```python
from build123d import *

# Parameters (mm, degrees)
SKIZZE2_W                        = 120
SKIZZE2_H                        = 39.364160046
AUFSATZ_LINEAR_AUSTRAGEN1_DEPTH  = 30
SKIZZE24_R                       = 1.55
SCHNITT_LINEAR_AUSTRAGEN4_DEPTH  = 130.805766806
SKIZZE46_R                       = 2.85
SCHNITT_LINEAR_AUSTRAGEN15_DEPTH = 10
SCHNITT_LINEAR_START             = -5
SCHNITT_LINEAR_AUSTRAGEN25_DEPTH = 2.7
LINEARES_MUSTER1_COUNT           = 5
LINEARES_MUSTER1_PITCH           = 20
SPIEGELN2_COPY_1_SKETCH_R        = 2.85
SPIEGELN2_COPY_1_DEPTH           = 10
SPIEGELN2_COPY_2_SKETCH_R        = 2.85
SPIEGELN2_COPY_2_DEPTH           = 10
SPIEGELN2_COPY_3_SKETCH_R        = 2.85
SPIEGELN2_COPY_3_DEPTH           = 10
SPIEGELN2_COPY_4_SKETCH_R        = 2.85
SPIEGELN2_COPY_4_DEPTH           = 10
SPIEGELN2_START                  = -5
SPIEGELN2_COPY_5_DEPTH           = 2.7
SPIEGELN2_COPY_6_DEPTH           = 2.7
SPIEGELN2_COPY_7_DEPTH           = 2.7
SPIEGELN2_COPY_8_DEPTH           = 2.7
SKIZZE51_R                       = 1.55
SCHNITT_LINEAR_AUSTRAGEN26_DEPTH = 130.805766806
SKIZZE67_R                       = 0.5
SCHNITT_LINEAR_AUSTRAGEN28_DEPTH = 16
SKIZZE68_R                       = 0.65
SCHNITT_LINEAR_AUSTRAGEN30_DEPTH = 16
SKIZZE70_R                       = 2
SCHNITT_LINEAR_AUSTRAGEN31_DEPTH = 6
ABSPALTEN3_OUTLINE_W             = 120
ABSPALTEN3_OUTLINE_H             = 39.364160046
ABSPALTEN3_OUTLINE_R             = 1.55
ABSPALTEN3_DEPTH                 = 15


# Read off the part's stored shape, not the designer's step: Abspalten3
with BuildPart() as part:
    # Skizze2 → Aufsatz-Linear austragen1 (new body)
    with BuildSketch(Plane.XY):
        with Locations((60, 19.682080023)):
            Rectangle(SKIZZE2_W, SKIZZE2_H)
    extrude(amount=AUFSATZ_LINEAR_AUSTRAGEN1_DEPTH)

    # Skizze24 → Schnitt-Linear austragen4 (cut, through all)
    with BuildSketch(Plane.XY.offset(30)):
        with Locations((20, 31.364160046)):
            Circle(SKIZZE24_R)
        with Locations((40, 31.364160046)):
            Circle(SKIZZE24_R)
        with Locations((60, 31.364160046)):
            Circle(SKIZZE24_R)
        with Locations((80, 31.364160046)):
            Circle(SKIZZE24_R)
        with Locations((100, 31.364160046)):
            Circle(SKIZZE24_R)
    schnitt_linear_austragen4 = extrude(amount=-SCHNITT_LINEAR_AUSTRAGEN4_DEPTH, mode=Mode.SUBTRACT)

    # Skizze46 → Schnitt-Linear austragen15 (cut)
    with BuildSketch(Plane(origin=(0, 0, 0), x_dir=(-1, 0, 0), z_dir=(0, 0, -1))):
        with Locations((-100, 31.364160046)):
            Circle(SKIZZE46_R)
    schnitt_linear_austragen15 = extrude(amount=-SCHNITT_LINEAR_AUSTRAGEN15_DEPTH, mode=Mode.SUBTRACT)

    # Skizze50 → Schnitt-Linear austragen25 (cut)
    with BuildSketch(Plane.XY.offset(30).offset(SCHNITT_LINEAR_START)):
        Polygon((97.15, 33.009608314), (97.15, 39.364160046), (102.85, 39.364160046), (102.85, 33.009608314), (102.85, 29.718711779), (100, 28.073263512), (97.15, 29.718711779), align=None)
    schnitt_linear_austragen25 = extrude(amount=-SCHNITT_LINEAR_AUSTRAGEN25_DEPTH, mode=Mode.SUBTRACT)

    # Lineares Muster1: Schnitt-Linear austragen15, Schnitt-Linear austragen25 ×5
    with Locations(*[(-i * LINEARES_MUSTER1_PITCH, 0, 0) for i in range(1, LINEARES_MUSTER1_COUNT)]):
        add(schnitt_linear_austragen15, mode=Mode.SUBTRACT)
        add(schnitt_linear_austragen25, mode=Mode.SUBTRACT)

    # Spiegeln2: Schnitt-Linear austragen15, Schnitt-Linear austragen25 across plane
    add(schnitt_linear_austragen15.mirror(Plane.ZX.offset(19.764160046)), mode=Mode.SUBTRACT)
    add(schnitt_linear_austragen25.mirror(Plane.ZX.offset(19.764160046)), mode=Mode.SUBTRACT)

    # Spiegeln2 copy 1 sketch → Spiegeln2 copy 1 (cut)
    with BuildSketch(Plane(origin=(-20, 39.528320093, 0), x_dir=(-1, 0, 0), z_dir=(0, 0, -1))):
        with Locations((-100, -31.364160046)):
            Circle(SPIEGELN2_COPY_1_SKETCH_R)
    extrude(amount=-SPIEGELN2_COPY_1_DEPTH, mode=Mode.SUBTRACT)

    # Spiegeln2 copy 2 sketch → Spiegeln2 copy 2 (cut)
    with BuildSketch(Plane(origin=(-40, 39.528320093, 0), x_dir=(-1, 0, 0), z_dir=(0, 0, -1))):
        with Locations((-100, -31.364160046)):
            Circle(SPIEGELN2_COPY_2_SKETCH_R)
    extrude(amount=-SPIEGELN2_COPY_2_DEPTH, mode=Mode.SUBTRACT)

    # Spiegeln2 copy 3 sketch → Spiegeln2 copy 3 (cut)
    with BuildSketch(Plane(origin=(-60, 39.528320093, 0), x_dir=(-1, 0, 0), z_dir=(0, 0, -1))):
        with Locations((-100, -31.364160046)):
            Circle(SPIEGELN2_COPY_3_SKETCH_R)
    extrude(amount=-SPIEGELN2_COPY_3_DEPTH, mode=Mode.SUBTRACT)

    # Spiegeln2 copy 4 sketch → Spiegeln2 copy 4 (cut)
    with BuildSketch(Plane(origin=(-80, 39.528320093, 0), x_dir=(-1, 0, 0), z_dir=(0, 0, -1))):
        with Locations((-100, -31.364160046)):
            Circle(SPIEGELN2_COPY_4_SKETCH_R)
    extrude(amount=-SPIEGELN2_COPY_4_DEPTH, mode=Mode.SUBTRACT)

    # Spiegeln2 copy 5 sketch → Spiegeln2 copy 5 (cut)
    with BuildSketch(Plane(origin=(-20, 39.528320093, 30), x_dir=(1, 0, 0), z_dir=(0, 0, 1)).offset(SPIEGELN2_START)):
        Polygon((97.15, -33.009608314), (97.15, -39.364160046), (102.85, -39.364160046), (102.85, -33.009608314), (102.85, -29.718711779), (100, -28.073263512), (97.15, -29.718711779), align=None)
    extrude(amount=-SPIEGELN2_COPY_5_DEPTH, mode=Mode.SUBTRACT)

    # Spiegeln2 copy 6 sketch → Spiegeln2 copy 6 (cut)
    with BuildSketch(Plane(origin=(-40, 39.528320093, 30), x_dir=(1, 0, 0), z_dir=(0, 0, 1)).offset(SPIEGELN2_START)):
        Polygon((97.15, -33.009608314), (97.15, -39.364160046), (102.85, -39.364160046), (102.85, -33.009608314), (102.85, -29.718711779), (100, -28.073263512), (97.15, -29.718711779), align=None)
    extrude(amount=-SPIEGELN2_COPY_6_DEPTH, mode=Mode.SUBTRACT)

    # Spiegeln2 copy 7 sketch → Spiegeln2 copy 7 (cut)
    with BuildSketch(Plane(origin=(-60, 39.528320093, 30), x_dir=(1, 0, 0), z_dir=(0, 0, 1)).offset(SPIEGELN2_START)):
        Polygon((97.15, -33.009608314), (97.15, -39.364160046), (102.85, -39.364160046), (102.85, -33.009608314), (102.85, -29.718711779), (100, -28.073263512), (97.15, -29.718711779), align=None)
    extrude(amount=-SPIEGELN2_COPY_7_DEPTH, mode=Mode.SUBTRACT)

    # Spiegeln2 copy 8 sketch → Spiegeln2 copy 8 (cut)
    with BuildSketch(Plane(origin=(-80, 39.528320093, 30), x_dir=(1, 0, 0), z_dir=(0, 0, 1)).offset(SPIEGELN2_START)):
        Polygon((97.15, -33.009608314), (97.15, -39.364160046), (102.85, -39.364160046), (102.85, -33.009608314), (102.85, -29.718711779), (100, -28.073263512), (97.15, -29.718711779), align=None)
    extrude(amount=-SPIEGELN2_COPY_8_DEPTH, mode=Mode.SUBTRACT)

    # Spiegeln3: Schnitt-Linear austragen4 across plane
    add(schnitt_linear_austragen4.mirror(Plane.ZX.offset(19.764160046)), mode=Mode.SUBTRACT)

    # Skizze51 → Schnitt-Linear austragen26 (cut, through all)
    with BuildSketch(Plane.XY.offset(30)):
        with Locations((5, 34.364160046)):
            Circle(SKIZZE51_R)
        with Locations((115, 5)):
            Circle(SKIZZE51_R)
    extrude(amount=-SCHNITT_LINEAR_AUSTRAGEN26_DEPTH, mode=Mode.SUBTRACT)

    # Skizze66 → Schnitt-Rotation5 (revolve, cut)
    with BuildSketch(Plane.XY.offset(15), mode=Mode.PRIVATE) as schnitt_rotation5_sk:
        Polygon((110, 19.682080023), (110, 21.182080023), (10, 22.682080023), (10, 19.682080023), align=None)
        Polygon((105, 19.682080023), (105, 23.757361257), (15, 25.107361257), (15, 19.682080023), align=None)
    revolve(schnitt_rotation5_sk.sketch.rotate(Axis((10, 19.682080023, 15), (1, 0, 0)), 180), axis=Axis((10, 19.682080023, 15), (1, 0, 0)), mode=Mode.SUBTRACT)

    # Skizze67 → Schnitt-Linear austragen28 (cut)
    with BuildSketch(Plane(origin=(120, 0, 0), x_dir=(0, 0, -1), z_dir=(1, 0, 0))):
        with Locations((-18.5, 19.764160046)):
            Circle(SKIZZE67_R)
    schnitt_linear_austragen28 = extrude(amount=-SCHNITT_LINEAR_AUSTRAGEN28_DEPTH, mode=Mode.SUBTRACT)

    # Spiegeln5: Schnitt-Linear austragen28 across plane
    add(schnitt_linear_austragen28.mirror(Plane.XY.offset(15)), mode=Mode.SUBTRACT)

    # Skizze68 → Schnitt-Linear austragen30 (cut)
    with BuildSketch(Plane.ZY):
        with Locations((10.25, 19.764160046)):
            Circle(SKIZZE68_R)
    extrude(amount=-SCHNITT_LINEAR_AUSTRAGEN30_DEPTH, mode=Mode.SUBTRACT)

    # Skizze70 → Schnitt-Linear austragen31 (cut)
    with BuildSketch(Plane.ZY):
        with Locations((10.25, 19.764160046)):
            Circle(SKIZZE70_R)
    extrude(amount=-SCHNITT_LINEAR_AUSTRAGEN31_DEPTH, mode=Mode.SUBTRACT)

    # Abspalten3 outline → Abspalten3 (cut)
    with BuildSketch(Plane.XY):
        with Locations((60, 19.682080023)):
            Rectangle(ABSPALTEN3_OUTLINE_W, ABSPALTEN3_OUTLINE_H)
        with Locations((115, 5)):
            Circle(ABSPALTEN3_OUTLINE_R, mode=Mode.SUBTRACT)
        with Locations((5, 34.364160046)):
            Circle(ABSPALTEN3_OUTLINE_R, mode=Mode.SUBTRACT)
        with Locations((20, 8.164160046)):
            Circle(ABSPALTEN3_OUTLINE_R, mode=Mode.SUBTRACT)
        with Locations((40, 8.164160046)):
            Circle(ABSPALTEN3_OUTLINE_R, mode=Mode.SUBTRACT)
        with Locations((60, 8.164160046)):
            Circle(ABSPALTEN3_OUTLINE_R, mode=Mode.SUBTRACT)
        with Locations((80, 8.164160046)):
            Circle(ABSPALTEN3_OUTLINE_R, mode=Mode.SUBTRACT)
        with Locations((100, 8.164160046)):
            Circle(ABSPALTEN3_OUTLINE_R, mode=Mode.SUBTRACT)
        with Locations((20, 31.364160046)):
            Circle(ABSPALTEN3_OUTLINE_R, mode=Mode.SUBTRACT)
        with Locations((40, 31.364160046)):
            Circle(ABSPALTEN3_OUTLINE_R, mode=Mode.SUBTRACT)
        with Locations((60, 31.364160046)):
            Circle(ABSPALTEN3_OUTLINE_R, mode=Mode.SUBTRACT)
        with Locations((80, 31.364160046)):
            Circle(ABSPALTEN3_OUTLINE_R, mode=Mode.SUBTRACT)
        with Locations((100, 31.364160046)):
            Circle(ABSPALTEN3_OUTLINE_R, mode=Mode.SUBTRACT)
    extrude(amount=ABSPALTEN3_DEPTH, mode=Mode.SUBTRACT)


solid = part.part
```
Design review of the part built by this model. Coordinates are the model's own, in mm. A direction names the side the tool comes from. Give positions to 0.01 mm unless a question says otherwise; leave off trailing zeros. Write each loop counter-clockwise with the first axis right and the second up, starting at its lowest first coordinate (ties: lowest second). Pieces come first, ordered by that corner, then holes.
(1) Clearance check with flat-ended pins moving along their axes: pin 1 Ø3.5 at (x, y) = (60, 8.16) entering from -Z; pin 2 Ø2 at (x, z) = (99, 23.5) entering from +Y; pin 3 Ø0.8 at (x, z) = (60, 23) entering from +Y. State where each tip first meets the part, or that it passes through.
Checked values:
pin 1: stops at z = 15
pin 2: stops at y = 29.23
pin 3: stops at y = 28.3
(2) Tool access review of faces 5 (the face through (38.59, 10.64, 23.67)), 6 (the face through (102.85, 34, 24)), 7 (the face through (107.465, 19.716, 16.538)), 8 (the face through (81.43, 30.77, 18.7)): name each direction out of +Z, -Z, +X, -X, +Y, -Y from which nothing blocks a thin tool from reaching the whole face with its end or side.
Checked values:
face 5: none
face 6: +Y
face 7: -Z
face 8: +Z, -Z
(3) Mouldability with a two-part tool opening along Y and no side actions: class faces 1 (the face through (40, 35, 22.3)), 2 (the face through (41.445, 28.908, 23.669)), 3 (the face through (81.445, 10.621, 23.669)), 4 (the face through (41.43, 30.77, 27.54)) as +Y half, -Y half, draft (parallel to the pull), parting line (faces both ways), or undercut.
Checked values:
face 1: draft
face 2: +Y half
face 3: undercut
face 4: undercut
(4) Add section D-D (x = 86). Give the boundary of the cut face in (y, z), and give its area (3 significant figures).
Checked values:
outline: (0, 15) - (15.32, 15) arc R4.36 cw to (24.04, 15) - (39.36, 15) - (39.36, 30) - (0, 30) - close
area: 561 mm2
(5) Add section C-C (z = 28.75). Give the number of separate pieces and of enclosed holes in the cut face, and give its area (3 significant figures).
Checked values:
separate pieces: 1
enclosed holes: 12
area: 4,630 mm2
(6) Wall thickness on line 1 along Y through (x, z) = (60, 20.5); line 2 along X through (y, z) = (30.5, 27.75); line 3 along Y through (x, z) = (20.5, 26.75): over which ranges is each line inside the solid? List them lowest first.
Checked values:
line 1: y = 0 to 6.61, 9.71 to 29.81, 32.91 to 39.36
line 2: x = 0 to 18.71, 21.29 to 38.71, 41.29 to 58.71, 61.29 to 78.71, 81.29 to 98.71, 101.29 to 120
line 3: y = 0 to 6.7, 9.63 to 29.9, 32.83 to 39.36
(7) Add section A-A (y = 5). Give the boundary of the cut face in (x, z).
Checked values:
outline: (0, 15) - (113.45, 15) - (113.45, 30) - (0, 30) - close; (116.55, 15) - (120, 15) - (120, 30) - (116.55, 30) - close; hole (17.15, 22.3) - (22.85, 22.3) - (22.85, 25) - (17.15, 25) - close; hole (37.15, 22.3) - (42.85, 22.3) - (42.85, 25) - (37.15, 25) - close; hole (57.15, 22.3) - (62.85, 22.3) - (62.85, 25) - (57.15, 25) - close; hole (77.15, 22.3) - (82.85, 22.3) - (82.85, 25) - (77.15, 25) - close; hole (97.15, 22.3) - (102.85, 22.3) - (102.85, 25) - (97.15, 25) - close
(8) Add section B-B (x = 115). Give the boundary of the cut face in (y, z), and give its area (3 significant figures).
Checked values:
outline: (0, 15) - (3.45, 15) - (3.45, 30) - (0, 30) - close; (6.55, 15) - (39.36, 15) - (39.36, 30) - (6.55, 30) - close; hole circle Ø1 at (19.76, 18.5)
area: 543 mm2
